Model file for the job. Use its own axes, mm. A direction names the side the tool comes from. Coordinates: 2 decimals unless noted, no trailing zeros. Order: outer loops, then holes, each group sorted by start corner. A loop starts at its lowest first (then second) coordinate and runs counter-clockwise, first axis right, second up. Notation, with made-up numbers: M 3.5,61.25 L 61.5,61.25 A31 cw 61.5,94.25 Z; hole C -16.5,-25.5 d1. An arc over 180 degrees is marked long. Return JSON: item names as keys, results as strings.
```python
from build123d import *

# Parameters (mm, degrees)
F0_W      = 40
F0_H      = 30
F1_DEPTH  = 10
F2_R      = 5
F3_T      = -2.5
F4_W      = 28
F4_H      = 2.5
F5_DEPTH  = 3
F6_W      = 32.3581136763
F6_H      = 60.2468792349
F7_DEPTH  = 25
F8_R      = 0.75
F9_DEPTH  = 0.75
F10_R     = 0.74999
F11_W     = 14
F11_H     = 2.5
F12_DEPTH = 0.2
F13_R     = 1
F15_W     = 15
F15_H     = 2.3
F16_DEPTH = 2.5


# Not quite as in the source:
# - a fillet or chamfer is up to 0.001 mm smaller than in the source, because OpenCascade refuses the exact size


with BuildPart() as f1:
    # F0 (on Top) → F1 (new body)
    with BuildSketch(Plane.XY):
        Rectangle(F0_W, F0_H)
    extrude(amount=-F1_DEPTH)

    # F2
    f2_edges = [f1.edges().sort_by_distance(p)[0] for p in [
        (20, 0, -10),
        (0, 15, -10),
        (-20, 0, -10),
        (0, -15, -10),
    ]]
    fillet(f2_edges, radius=F2_R)

    # F3
    f3_openings = [f1.faces().sort_by_distance(p)[0] for p in [
        (0, 0, 0),
    ]]
    offset(amount=F3_T, openings=f3_openings)

    # F4 (on face) → F5 (cut)
    with BuildSketch(Plane.XY):
        with Locations((0, 13.75)):
            Rectangle(F4_W, F4_H)
    extrude(amount=-F5_DEPTH, mode=Mode.SUBTRACT)

    # F6 (on Top) → F7 (cut)
    with BuildSketch(Plane.XY):
        with Locations((16.1790568382, -2.0559011027)):
            Rectangle(F6_W, F6_H)
    extrude(amount=-F7_DEPTH, mode=Mode.SUBTRACT)

    # F8 (on face) → F9 (cut)
    with BuildSketch(Plane.YZ.offset(-14)):
        with Locations((13.75, -1.5)):
            Circle(F8_R)
    extrude(amount=-F9_DEPTH, mode=Mode.SUBTRACT)

    # F10 (radius 0.75 in the source; OpenCascade refuses exactly that, so slightly less here)
    f10_edges = [f1.edges().sort_by_distance(p)[0] for p in [
        (-14.75, 13, -1.5),
    ]]
    fillet(f10_edges, radius=F10_R)

    # F11 (on face) → F12 (cut)
    with BuildSketch(Plane.XY.offset(-3)):
        with Locations((-7, 13.75)):
            Rectangle(F11_W, F11_H)
    extrude(amount=-F12_DEPTH, mode=Mode.SUBTRACT)

    # F13
    f13_edges = [f1.edges().sort_by_distance(p)[0] for p in [
        (-17, 15, 0),
        (-15.75, 12.5, 0),
        (-7, 15, -3.2),
        (-7, 12.5, -3.2),
    ]]
    fillet(f13_edges, radius=F13_R)

    # F14: F1 across plane


with BuildPart() as f1_1:
    add(f1.part)
    add(f1.part.mirror(Plane.YZ))

    # F15 (on face) → F16 (cut, through all)
    with BuildSketch(Plane.XZ.offset(15)):
        with Locations((0, -3.15)):
            Rectangle(F15_W, F15_H)
    extrude(amount=-F16_DEPTH, mode=Mode.SUBTRACT)


solid = f1_1.part
```
Item 1: Saw through at A-A (x = -6). Write the cut outline in (y, z), and give its area (3 significant figures).
Check result:
{"outline": "M -15,-5 A5 ccw -10,-10 L 10,-10 A5 ccw 15,-5 L 15,-4.2 A1 ccw 14,-3.2 L 13.5,-3.2 A1 ccw 12.5,-4.2 L 12.5,-5 A2.5 cw 10,-7.5 L -10,-7.5 A2.5 cw -12.5,-5 L -12.5,-4.3 L -15,-4.3 Z; M -15,-2 L -12.5,-2 L -12.5,0 L -15,0 Z", "area": "90.3 mm2"}
Item 2: Drop flat-ended pins along their axis: pin 1 Ø2 at (x, y) = (2.5, -13.5) entering from -Z; pin 2 Ø8 at (x, y) = (-6, 3) entering from +Z; pin 3 Ø1.5 at (x, z) = (-4.5, -3) entering from +Y. Give the stop position or say it passes through.
Check result:
{"pin 1": "stops at z = -9.33", "pin 2": "stops at z = -7.5", "pin 3": "stops at y = 14.89"}
Item 3: Saw through at B-B (y = 0.75). Write the cut outline in (x, z).
Check result:
{"outline": "M -20,-5 A5 ccw -15,-10 L 15,-10 A5 ccw 20,-5 L 20,0 L 17.5,0 L 17.5,-5 A2.5 cw 15,-7.5 L -15,-7.5 A2.5 cw -17.5,-5 L -17.5,0 L -20,0 Z"}
Item 4: Pull direction Z, two halves, no side cores. Call faces 4 (the flat face through (0, -12.5, -1)), 5 (the flat face through (0, -14, -2)), 6 (the flat face through (0, 0, -10)): +Z half, -Z half, draft (parallel to the pull), parting line (faces both ways), or undercut.
Check result:
{"face 4": "draft", "face 5": "undercut", "face 6": "-Z half"}
Item 5: Saw through at D-D (y = -12). Write the cut outline in (x, z).
Check result:
{"outline": "M -20,-5 A5 ccw -17,-9.58 L 17,-9.58 A5 ccw 20,-5 L 20,0 L 17.5,0 L 17.5,-5 A2.5 cw 17,-6.5 L -17,-6.5 A2.5 cw -17.5,-5 L -17.5,0 L -20,0 Z"}
Item 6: Wall check: line 1 (Y direction, x = 14.05, z = -1.5); line 2 (X direction, y = 6, z = -1.5); line 3 (Y direction, x = 14.5, z = -3.5). Give the ranges that are in metal, low to high.
Check result:
{"line 1": "y = -15 to -12.5, 12.5 to 13, 14.5 to 15", "line 2": "x = -20 to -17.5, 17.5 to 20", "line 3": "y = -15 to -12.5, 12.5 to 15"}
Item 7: 3-axis set-ups, long thin cutter, end or side, ignore diameter. For faces 1 (the cylindrical face through (-0.196, 14.715, -3.501)), 2 (the flat face through (0, -14, -4.3)), 3 (the flat face through (-17.5, 0, -2)): which of +Z, -Z, +X, -X, +Y, -Y reach the whole face in a straight line?
Check result:
{"face 1": "+Z, +Y", "face 2": "-Y", "face 3": "+Z"}
Item 8: Saw through at C-C (z = -5.5). Write the cut outline in (x, y), and give its area (3 significant figures).
Check result:
{"outline": "M -19.97,-14.97 L 19.97,-14.97 L 19.97,14.97 L -19.97,14.97 Z; hole M -17.45,-12.45 L 17.45,-12.45 L 17.45,12.45 L -17.45,12.45 Z", "area": "328 mm2"}
